For this review, take the finished solid that the model builds, in its own axes (mm). Face numbers are marked on the shaded views. A direction names the side the tool comes from. Give positions to 0.01 mm unless a question says otherwise; leave off trailing zeros. Loops run counter-clockwise (first coordinate to the right, second up) from the corner with the lowest first, then second, coordinate; pieces in that order, holes last. Notation, with made-up numbers: (-10, -28) -> (17, -28) arc R26 ccw to (17, 3) -> close; hole circle Ø3 at (84.5, 4). An arc over 180 degrees is marked (long way). Answer as CSV lines item,"result". Start each with the question number.
Item 1: For L1, parallel to Z at x = 0.65, y = -1.8; L2, parallel to Z at x = 1, y = 0.2; L3, parallel to X at y = -0.75, z = 18.5, list the stretches that pass through material, from the lowest coordinate up. Write a range as from..to.
Item 2: Clearance check with flat-ended pins moving along their axes: P1, Ø1.3, axis at x = 0.5, y = 0, coming from the -Z side; P2, Ø0.6, axis at y = -0.5, z = 1, coming from the -X side; P3, Ø3, axis at y = 1, z = 17.5, coming from the +X side. State where each tip first meets the part, or that it passes through.
Item 3: Add section A-A on y = 0. State the section outline as (x, z) points.
Item 4: Add section B-B on z = 10.25. State the section outline as (x, y) points, plus the area to 3 significant figures.
Item 5: Machinability: for the marked faces 1 and 2, which of the approach directions +Z, -Z, +X, -X, +Y, -Y give a long, thin tool a straight path to every point of the face, cutting with its end or side? Answer none if there is none.
Autodesk Inventor part; units mm, degrees
ref_plane "YZ Plane" through (0, 0, 0) normal (1, 0, 0) x (0, 1, 0)
ref_plane "XZ Plane" through (0, 0, 0) normal (0, 1, 0) x (-1, 0, 0)
ref_plane "XY Plane" through (0, 0, 0) normal (0, 0, 1) x (1, 0, 0)
sketch "スケッチ1" plane through (0, 0, 0) normal (0, 0, 1) x (1, 0, 0)
  circle A0 centre (0, 0) radius 2.75
  circle A1 centre (0, 0) radius 1.5
  dimension "d0" = 5.5
  dimension "d1" = 3
extrude "押し出し1" add sketch "スケッチ1" along normal blind 3
extrude "押し出し2" add sketch "スケッチ1" along normal blind 23 contours A1
chamfer "面取り1" distance 0.3 angle 45 1 edges at (-2.75, 0, 0)
sketch "スケッチ2" plane through (0, 0, 0) normal (0, 0, -1) x (-1, 0, 0)
  line L0 (0, -1.4434) -> (-1.25, -0.7217)
  line L1 (-1.25, -0.7217) -> (-1.25, 0.7217)
  line L2 (-1.25, 0.7217) -> (0, 1.4434)
  line L3 (0, 1.4434) -> (1.25, 0.7217)
  line L4 (1.25, 0.7217) -> (1.25, -0.7217)
  line L5 (1.25, -0.7217) -> (0, -1.4434)
  point P0 (0, 0)
  point P1 (0, 0)
  dimension "d9" = 2.5
extrude "押し出し3" cut sketch "スケッチ2" against normal blind 1.3
thread "ねじ1"
properties part number "キャップボルトM3×20" material "鋼"
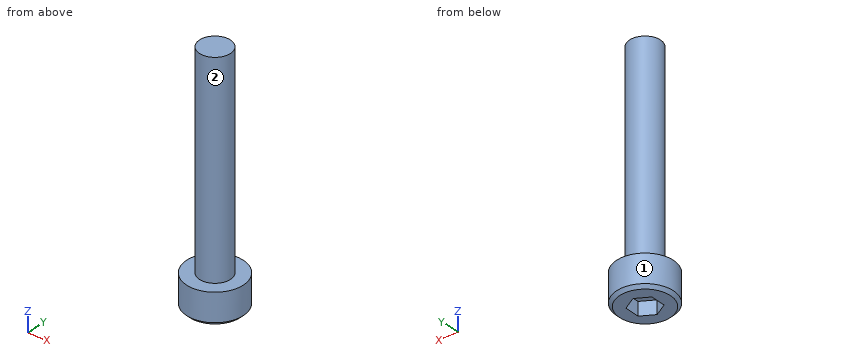
Computed values:
1,L1,"0..3"
1,L2,"1.3..23"
1,L3,"-1.3..1.3"
2,P1,"z = 1.3"
2,P2,"x = -2.74"
2,P3,"x = 1.5"
3,outline,"(-2.75, 0.3) -> (-2.45, 0) -> (-1.25, 0) -> (-1.25, 1.3) -> (1.25, 1.3) -> (1.25, 0) -> (2.45, 0) -> (2.75, 0.3) -> (2.75, 3) -> (1.5, 3) -> (1.5, 23) -> (-1.5, 23) -> (-1.5, 3) -> (-2.75, 3) -> close"
4,outline,"circle Ø3 at (0, 0)"
4,area,"7.07 mm²"
5,face 1,"+Z, -Z"
5,face 2,"+Z"
